```python
from build123d import *

# Parameters (mm, degrees)
SKETCH_1_W          = 220
SKETCH_1_H          = 144
SKETCH_1_R          = 1.6
SKETCH_1_R_2        = 1.6002032
EXTRUDE_1_DEPTH     = 2
CUT_EXTRUDE_1_DEPTH = 10
FILLET_1_R          = 10
CUT_EXTRUDE_2_DEPTH = 10
CUT_EXTRUDE_3_DEPTH = 10
SKETCH_8_R          = 1.6
CUT_EXTRUDE_4_DEPTH = 10
SKETCH_9_R          = 1.7
CUT_EXTRUDE_5_DEPTH = 10


with BuildPart() as part:
    # 草图1 → 凸台-拉伸1 (new body)
    with BuildSketch(Plane.XY):
        with Locations((60, -41.5)):
            Rectangle(SKETCH_1_W, SKETCH_1_H)
        with Locations((135, 11.5)):
            Circle(SKETCH_1_R, mode=Mode.SUBTRACT)
        with Locations((135, -12.5)):
            Circle(SKETCH_1_R, mode=Mode.SUBTRACT)
        with Locations((105, 11.5)):
            Circle(SKETCH_1_R, mode=Mode.SUBTRACT)
        with Locations((105, -12.5)):
            Circle(SKETCH_1_R, mode=Mode.SUBTRACT)
        with Locations((135, -70.5)):
            Circle(SKETCH_1_R, mode=Mode.SUBTRACT)
        with Locations((135, -94.5)):
            Circle(SKETCH_1_R, mode=Mode.SUBTRACT)
        with Locations((105, -70.5)):
            Circle(SKETCH_1_R, mode=Mode.SUBTRACT)
        with Locations((105, -94.5)):
            Circle(SKETCH_1_R, mode=Mode.SUBTRACT)
        with Locations((15, 11.5)):
            Circle(SKETCH_1_R, mode=Mode.SUBTRACT)
        with Locations((-15, 11.5)):
            Circle(SKETCH_1_R, mode=Mode.SUBTRACT)
        with Locations((15, -12.5)):
            Circle(SKETCH_1_R, mode=Mode.SUBTRACT)
        with Locations((-15, -12.5)):
            Circle(SKETCH_1_R, mode=Mode.SUBTRACT)
        with Locations((15, -70.5)):
            Circle(SKETCH_1_R, mode=Mode.SUBTRACT)
        with Locations((-15, -70.5)):
            Circle(SKETCH_1_R, mode=Mode.SUBTRACT)
        with Locations((15, -94.5)):
            Circle(SKETCH_1_R, mode=Mode.SUBTRACT)
        with Locations((-15, -94.5)):
            Circle(SKETCH_1_R, mode=Mode.SUBTRACT)
        with Locations((24.487307595, -8.49993523)):
            Circle(SKETCH_1_R_2, mode=Mode.SUBTRACT)
        with Locations((85.487429515, -8.49993523)):
            Circle(SKETCH_1_R_2, mode=Mode.SUBTRACT)
        with Locations((24.487307595, -74.50006731)):
            Circle(SKETCH_1_R, mode=Mode.SUBTRACT)
        with Locations((85.487429515, -74.50006731)):
            Circle(SKETCH_1_R_2, mode=Mode.SUBTRACT)
        with Locations((76.987299975, -19.5000762)):
            Circle(SKETCH_1_R, mode=Mode.SUBTRACT)
        with Locations((76.987299975, -63.5000762)):
            Circle(SKETCH_1_R, mode=Mode.SUBTRACT)
        with Locations((32.987299975, -63.5000762)):
            Circle(SKETCH_1_R, mode=Mode.SUBTRACT)
        with Locations((32.987299975, -19.5000762)):
            Circle(SKETCH_1_R, mode=Mode.SUBTRACT)
    extrude(amount=EXTRUDE_1_DEPTH)

    # 草图4 → 切除-拉伸1 (cut)
    with BuildSketch(Plane.XY.offset(2)):
        with BuildLine():
            Line((92.5, -28.5), (127.5, -28.5))
            ThreePointArc((127.5, -28.5), (140.5, -41.5), (127.5, -54.5))
            Line((127.5, -54.5), (92.5, -54.5))
            ThreePointArc((92.5, -54.5), (79.5, -41.5), (92.5, -28.5))
        make_face()
    extrude(amount=-CUT_EXTRUDE_1_DEPTH, mode=Mode.SUBTRACT)

    # 圆角1
    fillet_1_edges = [part.edges().sort_by_distance(p)[0] for p in [
        (-50, -113.5, 1),
        (-50, 30.5, 1),
        (170, 30.5, 1),
        (170, -113.5, 1),
    ]]
    fillet(fillet_1_edges, radius=FILLET_1_R)

    # 草图5 → 切除-拉伸2 (cut)
    with BuildSketch(Plane.XY.offset(2)):
        with BuildLine():
            Line((5, -32.5), (60, -32.5))
            ThreePointArc((60, -32.5), (69, -41.5), (60, -50.5))
            Line((60, -50.5), (5, -50.5))
            ThreePointArc((5, -50.5), (-4, -41.5), (5, -32.5))
        make_face()
    extrude(amount=-CUT_EXTRUDE_2_DEPTH, mode=Mode.SUBTRACT)

    # 草图6 → 切除-拉伸3 (cut)
    with BuildSketch(Plane.XY.offset(2)):
        with BuildLine():
            Line((35, 8.5), (75, 8.5))
            ThreePointArc((75, 8.5), (81, 2.5), (75, -3.5))
            Line((75, -3.5), (35, -3.5))
            ThreePointArc((35, -3.5), (29, 2.5), (35, 8.5))
        make_face()
        with BuildLine():
            Line((35, -91.5), (75, -91.5))
            ThreePointArc((75, -91.5), (81, -85.5), (75, -79.5))
            Line((75, -79.5), (35, -79.5))
            ThreePointArc((35, -79.5), (29, -85.5), (35, -91.5))
        make_face()
    extrude(amount=-CUT_EXTRUDE_3_DEPTH, mode=Mode.SUBTRACT)

    # 草图8 → 切除-拉伸4 (cut)
    with BuildSketch(Plane.XY.offset(2)):
        with Locations((-40, -32)):
            Circle(SKETCH_8_R)
        with Locations((-40, -51)):
            Circle(SKETCH_8_R)
        with BuildLine():
            Line((-29, -26.5), (-29, -56.5))
            ThreePointArc((-29, -56.5), (-32, -59.5), (-35, -56.5))
            Line((-35, -56.5), (-35, -26.5))
            ThreePointArc((-35, -26.5), (-32, -23.5), (-29, -26.5))
        make_face()
    extrude(amount=-CUT_EXTRUDE_4_DEPTH, mode=Mode.SUBTRACT)

    # 草图9 → 切除-拉伸5 (cut)
    with BuildSketch(Plane.XY.offset(2)):
        with Locations((-25, -70.5)):
            Circle(SKETCH_9_R)
        with Locations((-25, -12.5)):
            Circle(SKETCH_9_R)
    extrude(amount=-CUT_EXTRUDE_5_DEPTH, mode=Mode.SUBTRACT)


solid = part.part
```
Geometry check sheet. Reference: the model listing, model coordinates, mm. A direction names the side the tool comes from. Coordinates: 2 decimals unless noted, no trailing zeros. Write each loop counter-clockwise with the first axis right and the second up, starting at its lowest first coordinate (ties: lowest second). Pieces come first, ordered by that corner, then holes. Notation, with made-up numbers: (33.5, 31.25) -> (73.5, 31.25) arc R23 cw to (73.5, 39.25) -> close; hole circle Ø9 at (63.5, -29). An arc over 180 degrees is marked (long way). Use CSV: the item, a comma, the result in double quotes. Start each with the question number.
Item 1: Set-up check for faces 4 (the cylindrical face through (166.99, 27.65, 1.01)), 5 (the cylindrical face through (81, 2.6, 1)): record each of +Z, -Z, +X, -X, +Y, -Y from which the full face is reachable in a straight line by a thin tool's end or side.
Item 2: Mould release check, pull along X, two halves, no side actions. Record for faces 1 (the cylindrical face through (-47.15, -110.49, 1.01)), 2 (the cylindrical face through (29, 2.4, 1)), 3 (the cylindrical face through (166.99, -110.65, 1.01)): released by +X, released by -X, zero draft, split by the parting line, or undercut.
Item 3: Cross-section at B-B, the plane z = 1.3. State how many separate pieces and enclosed holes the cut face has, plus the area to 3 significant figures.
Item 4: Thickness scan on line 1 (Y direction, x = -15, z = 0.55); line 2 (X direction, y = -94.5, z = 0.7); line 3 (Y direction, x = 105, z = 1.05). Record the ranges inside material, lowest first.
Item 5: Depth check by flat-ended pin: pin 1 Ø3 at (x, y) = (-15, -70.5) entering from -Z. Enter the tip coordinate at first touch or a pass-through.
Item 6: Cross-section at A-A, the plane x = 131. Record the cut outline in (y, z).
Answers:
1,face 4,"+Z, -Z, +X, +Y"
1,face 5,"+Z, -Z"
2,face 1,"released by -X"
2,face 2,"undercut"
2,face 3,"released by +X"
3,separate pieces,"1"
3,enclosed holes,"33"
3,area,"27,300 mm^2"
4,line 1,"-113.5 to -96.1, -92.9 to -72.1, -68.9 to -14.1, -10.9 to 9.9, 13.1 to 30.5"
4,line 2,"-50 to -16.6, -13.4 to 13.4, 16.6 to 103.4, 106.6 to 133.4, 136.6 to 170"
4,line 3,"-113.5 to -96.1, -92.9 to -72.1, -68.9 to -54.5, -28.5 to -14.1, -10.9 to 9.9, 13.1 to 30.5"
5,pin 1,"through"
6,outline,"(-113.5, 0) -> (-54.02, 0) -> (-54.02, 2) -> (-113.5, 2) -> close; (-28.98, 0) -> (30.5, 0) -> (30.5, 2) -> (-28.98, 2) -> close"
